from build123d import *

# Parameters (mm, degrees)
F0_W     = 10
F0_H     = 25
F0_W_2   = 8
F0_H_2   = 23
F1_DEPTH = 5
F2_W     = 12
F2_H     = 27
F2_W_2   = 10
F2_H_2   = 25
F2_W_3   = 8
F2_H_3   = 23
F3_DEPTH = 0.5
F4_W     = 12
F4_H     = 27
F4_W_2   = 10
F4_H_2   = 25
F4_W_3   = 8
F4_H_3   = 23
F5_DEPTH = 0.5
F7_W     = 12
F7_H     = 1
F8_DEPTH = 25
F9_R     = 1


with BuildPart() as f1:
    # F0 (on Front) → F1 (new body)
    with BuildSketch(Plane.XZ):
        Rectangle(F0_W, F0_H)
        Rectangle(F0_W_2, F0_H_2, mode=Mode.SUBTRACT)
    extrude(amount=F1_DEPTH)

    # F2 (on face) → F3 (join)
    with BuildSketch(Plane(origin=(0, 0, 0), x_dir=(-1, 0, 0), z_dir=(0, 1, 0))):
        Rectangle(F2_W, F2_H)
        Rectangle(F2_W_2, F2_H_2, mode=Mode.SUBTRACT)
        Rectangle(F2_W_2, F2_H_2)
        Rectangle(F2_W_3, F2_H_3, mode=Mode.SUBTRACT)
    extrude(amount=F3_DEPTH)

    # F4 (on face) → F5 (join)
    with BuildSketch(Plane.XZ.offset(5)):
        Rectangle(F4_W, F4_H)
        Rectangle(F4_W_2, F4_H_2, mode=Mode.SUBTRACT)
        Rectangle(F4_W_2, F4_H_2)
        Rectangle(F4_W_3, F4_H_3, mode=Mode.SUBTRACT)
    extrude(amount=F5_DEPTH)

    # F7 (on face) → F8 (cut)
    with BuildSketch(Plane(origin=(0, 0.5, 0), x_dir=(-1, 0, 0), z_dir=(0, 1, 0))):
        with Locations((0, 13)):
            Rectangle(F7_W, F7_H)
    extrude(amount=-F8_DEPTH, mode=Mode.SUBTRACT)

    # F9
    f9_edges = [f1.edges().sort_by_distance(p)[0] for p in [
        (-5, -2.5, 12.5),
        (5, -2.5, 12.5),
        (-5, -2.5, -12.5),
        (5, -2.5, -12.5),
    ]]
    fillet(f9_edges, radius=F9_R)


solid = f1.part
The model under review builds one solid part; all positions refer to its coordinate system, in mm. A direction names the side the tool comes from. Coordinates: 2 decimals unless noted, no trailing zeros. Order: outer loops, then holes, each group sorted by start corner. A loop starts at its lowest first (then second) coordinate and runs counter-clockwise, first axis right, second up. Notation, with made-up numbers: (-3, 21.5) -> (32, 21.5) arc R21 ccw to (32, 54.5) -> close; hole circle Ø5 at (76, 24.25). An arc over 180 degrees is marked (long way). Answer in a Markdown table with one row per item.
(1) Insertion check: pin 1 (3 mm diameter, centred on x = 0, y = -3, fed in from -Z); pin 2 (3.5 mm diameter, centred on x = -0.5, z = 3.5, fed in from +Y); pin 3 (2.5 mm diameter, centred on y = -3.5, z = 4, fed in from +X). Each pin has a flat end and moves straight along its axis. Give the tip position at first contact, or say it passes through.
Answers:
| item | result |
|---|---|
| pin 1 | z = -12.5 |
| pin 2 | through |
| pin 3 | x = 5 |
(2) Consider section C-C (y = -0.75). Write out the cut boundary in (x, z).
Answers:
| item | result |
|---|---|
| outline | (-5, -11.5) arc R1 ccw to (-4, -12.5) -> (4, -12.5) arc R1 ccw to (5, -11.5) -> (5, 11.5) arc R1 ccw to (4, 12.5) -> (-4, 12.5) arc R1 ccw to (-5, 11.5) -> close; hole (-4, -11.5) -> (4, -11.5) -> (4, 11.5) -> (-4, 11.5) -> close |
(3) Consider section B-B (x = 0.75). Write out the cut boundary in (y, z).
Answers:
| item | result |
|---|---|
| outline | (-5.5, -13.5) -> (-5, -13.5) -> (-5, -12.5) -> (0, -12.5) -> (0, -13.5) -> (0.5, -13.5) -> (0.5, -11.5) -> (-5.5, -11.5) -> close; (-5.5, 11.5) -> (0.5, 11.5) -> (0.5, 12.5) -> (-5.5, 12.5) -> close |
(4) The part is to be moulded in two halves that separate along X. For faces 1 (the flat face through (5, -2, 0)), 2 (the flat face through (0, -2, -11.5)), 3 (the flat face through (0, -2, 11.5)), 4 (the flat face through (0, -2, -12.5)), say which applies: +X half, -X half, draft (parallel to the pull), parting line (faces both ways), or undercut.
Answers:
| item | result |
|---|---|
| face 1 | +X half |
| face 2 | undercut |
| face 3 | undercut |
| face 4 | draft |
(5) Consider section A-A (z = -1.25). Write out the cut boundary in (x, y).
Answers:
| item | result |
|---|---|
| outline | (-6, -5.5) -> (-4, -5.5) -> (-4, 0.5) -> (-6, 0.5) -> (-6, 0) -> (-5, 0) -> (-5, -5) -> (-6, -5) -> close; (4, -5.5) -> (6, -5.5) -> (6, -5) -> (5, -5) -> (5, 0) -> (6, 0) -> (6, 0.5) -> (4, 0.5) -> close |
(6) Machinability: for faces 5 (the cylindrical face through (-4.715, -2.535, -12.199)), 6 (the cylindrical face through (4.699, -2.535, -12.215)), 7 (the flat face through (4, -2, 0)), 8 (the flat face through (-5, -2, 0)), which of the approach directions +Z, -Z, +X, -X, +Y, -Y give a long, thin tool a straight path to every point of the face, cutting with its end or side? Answer none if there is none.
Answers:
| item | result |
|---|---|
| face 5 | -Z, -X |
| face 6 | -Z, +X |
| face 7 | +Y, -Y |
| face 8 | +Z, -Z, -X |
(7) Wall thickness on line 1 along Z through (x, y) = (1.25, -2.6); line 2 along X through (y, z) = (-4.75, 5.5); line 3 along Y through (x, z) = (-5.5, 6.75): over which ranges is each line inside the solid? List them lowest first.
Answers:
| item | result |
|---|---|
| line 1 | -12.5 to -11.5, 11.5 to 12.5 |
| line 2 | -5 to -4, 4 to 5 |
| line 3 | -5.5 to -5, 0 to 0.5 |
